```python
from build123d import *

# Parameters (mm, degrees)
ESQUISSE1_R             = 2.4
ESQUISSE1_R_2           = 2.16514488
BOSS_EXTRU_1_DEPTH      = 1.92
ENL_V_MAT_EXTRU_1_DEPTH = 0.72
CONG_6_R                = 0.36
ESQUISSE3_R             = 1.2
BOSS_EXTRU_2_DEPTH      = 7.2
CONG_7_R                = 0.6


with BuildPart() as part:
    # Esquisse1 → Boss.-Extru.1 (new body)
    # profile 1 of 3: a face of its own
    with BuildSketch(Plane.XY):
        Circle(ESQUISSE1_R)
        Circle(ESQUISSE1_R_2, mode=Mode.SUBTRACT)
    # profile 2 of 3: a face of its own
    with BuildSketch(Plane.XY):
        Circle(ESQUISSE1_R_2)
        Polygon((-0.258, -1.318102798), (-0.258, -0.258), (-1.224, -0.258), (-1.224, 0.258), (-0.258, 0.258), (-0.258, 1.318102798), (0.258, 1.318102798), (0.258, 0.258), (1.224, 0.258), (1.224, -0.258), (0.258, -0.258), (0.258, -1.318102798), align=None, mode=Mode.SUBTRACT)
    # profile 3 of 3: a face of its own
    with BuildSketch(Plane.XY):
        Polygon((-0.258, -0.258), (-1.224, -0.258), (-1.224, 0.258), (-0.258, 0.258), (-0.258, 1.318102798), (0.258, 1.318102798), (0.258, 0.258), (1.224, 0.258), (1.224, -0.258), (0.258, -0.258), (0.258, -1.318102798), (-0.258, -1.318102798), align=None)
    extrude(amount=BOSS_EXTRU_1_DEPTH)

    # Esquisse2 → Enlèv. mat.-Extru.1 (cut)
    with BuildSketch(Plane(origin=(0, 0, 0), x_dir=(-1, 0, 0), z_dir=(0, 0, -1))):
        Polygon((0, -1.224), (0, 0), (-1.224, 0), (-1.224, -0.258), (-0.258, -0.258), (-0.258, -1.224), align=None)
        Polygon((0, 0), (0, 1.224), (-0.258, 1.224), (-0.258, 0.258), (-1.224, 0.258), (-1.224, 0), align=None)
        Polygon((0.258, 1.224), (0, 1.224), (0, 0), (1.224, 0), (1.224, 0.258), (0.258, 0.258), align=None)
        Polygon((1.224, 0), (0, 0), (0, -1.224), (0.258, -1.224), (0.258, -0.258), (1.224, -0.258), align=None)
    extrude(amount=-ENL_V_MAT_EXTRU_1_DEPTH, mode=Mode.SUBTRACT)

    # Congé6
    cong_6_edges = [part.edges().sort_by_distance(p)[0] for p in [
        (0, -1.224, 0.72),
        (1.224, 0, 0.72),
        (-1.224, 0, 0.72),
        (0, 1.224, 0.72),
    ]]
    fillet(cong_6_edges, radius=CONG_6_R)

    # Esquisse3 → Boss.-Extru.2 (add)
    with BuildSketch(Plane.XY.offset(1.92)):
        Circle(ESQUISSE3_R)
    extrude(amount=BOSS_EXTRU_2_DEPTH)

    # Congé7
    cong_7_edges = [part.edges().sort_by_distance(p)[0] for p in [
        (-2.4, 0, 0),
    ]]
    fillet(cong_7_edges, radius=CONG_7_R)


solid = part.part
```
Could you check a few things on this model? Use its own coordinates, in mm. A direction names the side the tool comes from. Round coordinates to 2 decimals unless told otherwise and drop trailing zeros. Loops run counter-clockwise (first coordinate to the right, second up) from the corner with the lowest first, then second, coordinate; pieces in that order, holes last. Notation, with made-up numbers: M 23.5,77 L 27.5,77 A17 ccw 27.5,100 Z; hole C 39.5,-29 d5. An arc over 180 degrees is marked long. Write item = value, one per line.
1. Which directions (+Z, -Z, +X, -X, +Y, -Y) give clear straight access to the entire face, cutting with the end or side of a thin tool? Please do faces 1 (the face through (1.29, 2.024, 1.251)), 2 (the face through (-1, 1, 1.92)).
Results below:
face_1 = +Z, -Z
face_2 = +Z
2. I want a section at A-A, the plane x = 0. Write out the boundary of the cut face in (y, z), and give its area (3 significant figures).
Results below:
outline = M -2.4,0.6 A0.6 ccw -1.8,0 L -1.22,0 L -1.22,0.36 A0.36 cw -0.86,0.72 L 0.86,0.72 A0.36 cw 1.22,0.36 L 1.22,0 L 1.8,0 A0.6 ccw 2.4,0.6 L 2.4,1.92 L 1.2,1.92 L 1.2,9.12 L -1.2,9.12 L -1.2,1.92 L -2.4,1.92 Z
area = 24.6 mm²
3. I need wall thicknesses on probe 1 along Z at (x, y) = (1.15, 0.85); probe 2 along X at (y, z) = (0.05, 2.5); probe 3 along Y at (x, z) = (0.2, 0.5). Which ranges of each line are inside material? Lowest first, please.
Results below:
probe_1 = 0 to 1.92
probe_2 = -1.2 to 1.2
probe_3 = -2.38 to -1.2, 1.2 to 2.38
4. Thinking about a two-plate mould opening in X: for faces 3 (the face through (0, 0, 9.12)), 4 (the face through (0.65, 1.01, 5.47)), 5 (the face through (0, 0, 0.72)), which applies, +X half, -X half, draft (parallel to the pull), parting line (faces both ways), or undercut?
Results below:
face_3 = draft
face_4 = parting line
face_5 = undercut
5. Will these pins go through, and if not, where does the flat tip stop? P1, Ø1, axis at x = 1.5, z = 2, coming from the -Y side; P2, Ø1, axis at x = -1.5, y = 2, coming from the +Z side; P3, Ø1, axis at y = -0.5, z = 4.5, coming from the +X side.
Results below:
P1 = -2.18
P2 = 1.92
P3 = 1.2
6. I want a section at C-C, the plane z = 5.25. Write out the boundary of the cut face in (x, y).
Results below:
outline = C 0,0 d2.4
